from build123d import *

# Parameters (mm, degrees)
BOSS_EXTRUDE1_DEPTH = 3
SKETCH3_W           = 3
SKETCH3_H           = 12
CUT_EXTRUDE1_DEPTH  = 6


with BuildPart() as part:
    # Sketch2 → Boss-Extrude1 (new body)
    with BuildSketch(Plane.XY):
        Polygon((-65.471428571, 3), (-53.786813187, 3), (-53.786813187, 6), (-41.786813187, 6), (-41.786813187, 3), (-29.879120879, 3), (-29.879120879, 6), (-17.879120879, 6), (-17.879120879, 3), (-5.971428571, 3), (-5.971428571, 6), (6.028571429, 6), (6.028571429, 3), (17.936263736, 3), (17.936263736, 6), (29.936263736, 6), (29.936263736, 3), (41.843956044, 3), (41.843956044, 6), (53.843956044, 6), (53.843956044, 3), (65.528571429, 3), (65.528571429, 69), (53.815384615, 69), (53.815384615, 66), (41.872527473, 66), (41.872527473, 69), (29.907692308, 69), (29.907692308, 66), (17.964835165, 66), (17.964835165, 69), (6, 69), (6, 66), (-5.942857143, 66), (-5.942857143, 69), (-17.907692308, 69), (-17.907692308, 66), (-29.850549451, 66), (-29.850549451, 69), (-41.815384615, 69), (-41.815384615, 66), (-53.758241758, 66), (-53.758241758, 69), (-65.471428571, 69), align=None)
    extrude(amount=BOSS_EXTRUDE1_DEPTH)

    # Sketch3 → Cut-Extrude1 (cut)
    with BuildSketch(Plane.XY.offset(3)):
        with Locations((-63.971428571, 60)):
            Rectangle(SKETCH3_W, SKETCH3_H)
        with Locations((-63.971428571, 12)):
            Rectangle(SKETCH3_W, SKETCH3_H)
        with Locations((64.028571429, 36)):
            Rectangle(SKETCH3_W, SKETCH3_H)
        with Locations((64.028571429, 12)):
            Rectangle(SKETCH3_W, SKETCH3_H)
        with Locations((-63.971428571, 36)):
            Rectangle(SKETCH3_W, SKETCH3_H)
        with Locations((64.028571429, 60)):
            Rectangle(SKETCH3_W, SKETCH3_H)
    extrude(amount=-CUT_EXTRUDE1_DEPTH, mode=Mode.SUBTRACT)


solid = part.part
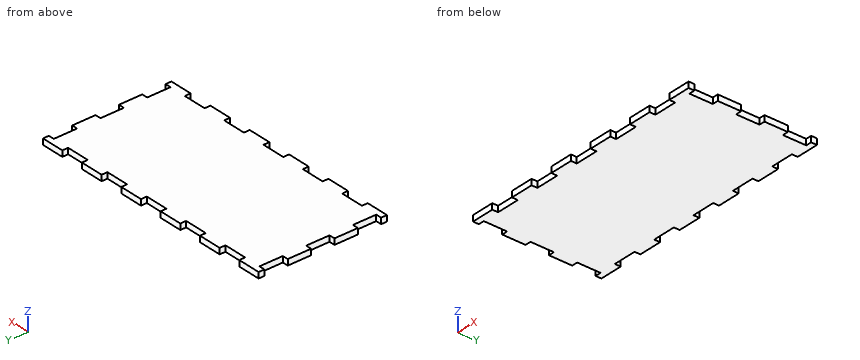
Build history of the part. All positions in model axes, mm. Coordinates: 2 decimals unless noted, no trailing zeros. Order: outer loops, then holes, each group sorted by start corner. A loop starts at its lowest first (then second) coordinate and runs counter-clockwise, first axis right, second up. Notation, with made-up numbers: M 9,76 L 57,76 A16 ccw 57,94 Z; hole C 88.25,6.25 d2. An arc over 180 degrees is marked long. One line per question, with ' | ' between items. Start each with the question number.
Q1. Saw through at A-A (y = 62). List the corners of the cut face in (x, z).
Q2. Probe L1, parallel to Y at x = -3.5, z = 0.6; L2, parallel to X at y = 63.5, z = 1.5. List the from-to ranges inside material, lowest first. Write a range as from..to.
Q3. Flat gauge pins, fed straight in: pin 1 Ø1.5 at (x, z) = (-48, 1.5) entering from -Y; pin 2 Ø0.9 at (x, z) = (25, 2) entering from +Y; pin 3 Ø1.5 at (x, y) = (38, 15.5) entering from -Z; pin 4 Ø0.9 at (y, z) = (33.5, 1.5) entering from -X. Where does each tip first touch, or does it go through?
Q4. Saw through at B-B (x = 4). List the corners of the cut face in (y, z).
Check values:
1) outline: M -62.47,0 L 62.53,0 L 62.53,3 L -62.47,3 Z
2) L1: y = 6..66 | L2: x = -62.47..62.53
3) pin 1: stops at y = 6 | pin 2: stops at y = 66 | pin 3: stops at z = 0 | pin 4: stops at x = -62.47
4) outline: M 6,0 L 66,0 L 66,3 L 6,3 Z
